Source: CAD feature listing. Evaluate the final solid. Frame: model axes, mm. Face numbers are marked on the shaded views. A direction names the side the tool comes from. Give positions to 0.01 mm unless a question says otherwise; leave off trailing zeros. Write each loop counter-clockwise with the first axis right and the second up, starting at its lowest first coordinate (ties: lowest second). Pieces come first, ordered by that corner, then holes. Notation, with made-up numbers: (48, -22) -> (104, -22) arc R23 ccw to (104, 11) -> close; hole circle Ø11 at (75, 54.25). An arc over 180 degrees is marked (long way). Write item = value, one per line.
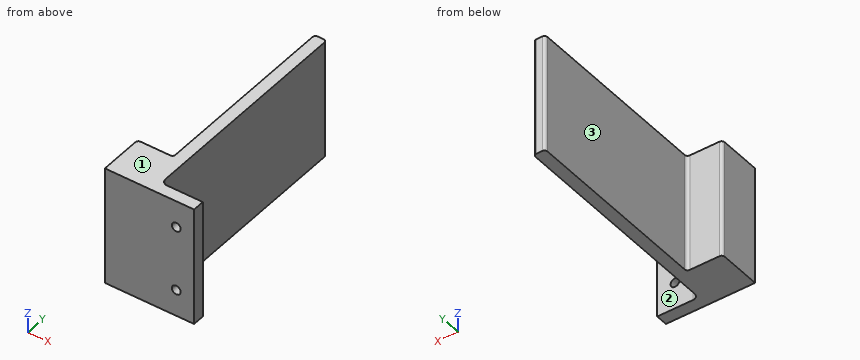
from build123d import *

# Parameters (mm, degrees)
PAD_DEPTH    = 40
FILLET_R     = 1
FILLET001_R  = 1
FILLET002_R  = 2
FILLET003_R  = 1
FILLET004_R  = 1
SKETCH001_R  = 1.5
POCKET_DEPTH = 5


with BuildPart() as part:
    # Sketch → Pad (new body)
    with BuildSketch(Plane.XY):
        Polygon((0, 0), (0, 15), (12, 15), (12, 80), (16, 80), (16, 4), (30, 4), (30, 0), align=None)
    extrude(amount=PAD_DEPTH)

    # Fillet
    fillet_edges = [part.edges().sort_by_distance(p)[0] for p in [
        (12, 80, 20),
    ]]
    fillet(fillet_edges, radius=FILLET_R)

    # Fillet001
    fillet001_edges = [part.edges().sort_by_distance(p)[0] for p in [
        (16, 80, 20),
    ]]
    fillet(fillet001_edges, radius=FILLET001_R)

    # Fillet002
    fillet002_edges = [part.edges().sort_by_distance(p)[0] for p in [
        (16, 4, 20),
    ]]
    fillet(fillet002_edges, radius=FILLET002_R)

    # Fillet003
    fillet003_edges = [part.edges().sort_by_distance(p)[0] for p in [
        (0, 15, 20),
    ]]
    fillet(fillet003_edges, radius=FILLET003_R)

    # Fillet004
    fillet004_edges = [part.edges().sort_by_distance(p)[0] for p in [
        (12, 15, 20),
    ]]
    fillet(fillet004_edges, radius=FILLET004_R)

    # Sketch001 (on Face12 of Fillet004) → Pocket (cut)
    with BuildSketch(Plane(origin=(0, 4, 0), x_dir=(-1, 0, 0), z_dir=(0, 1, 0))):
        with Locations((-24, 31)):
            Circle(SKETCH001_R)
        with Locations((-24, 9)):
            Circle(SKETCH001_R)
    extrude(amount=-POCKET_DEPTH, mode=Mode.SUBTRACT)


solid = part.part
1) Cut plane D-D (x = 9). Return the cut outline in (y, z), then the cut area to 3 significant figures.
Computed:
outline = (0, 0) -> (15, 0) -> (15, 40) -> (0, 40) -> close
area = 600 mm²
2) Material intervals for L1, parallel to Z at x = 24, y = 2.7; L2, parallel to Y at x = 20.5, z = 23.5; L3, parallel to Y at x = 7, z = 9.5, sorted ascending.
Computed:
L1 = 0 to 7.5, 10.5 to 29.5, 32.5 to 40
L2 = 0 to 4
L3 = 0 to 15
3) Cut plane B-B (z = 31). Return the cut outline in (x, y).
Computed:
outline = (0, 0) -> (22.5, 0) -> (22.5, 4) -> (18, 4) arc R2 cw to (16, 6) -> (16, 79) arc R1 ccw to (15, 80) -> (13, 80) arc R1 ccw to (12, 79) -> (12, 16) arc R1 cw to (11, 15) -> (1, 15) arc R1 ccw to (0, 14) -> close; (25.5, 0) -> (30, 0) -> (30, 4) -> (25.5, 4) -> close
4) Contact query for flat-ended pins moving along their axis: pin 1 (12 mm diameter, centred on y = 34, z = 21.5, fed in from +X); pin 2 (8 mm diameter, centred on x = 14.5, z = 13.5, fed in from -Y); pin 3 (11 mm diameter, centred on x = 5, z = 23, fed in from +Y); pin 4 (3.5 mm diameter, centred on x = 24, z = 15.5, fed in from +Y). Output: stop coordinate, or through.
Computed:
pin_1 = 16
pin_2 = 0
pin_3 = 15
pin_4 = 4
5) Cut plane A-A (x = 24). Return the cut outline in (y, z).
Computed:
outline = (0, 0) -> (4, 0) -> (4, 7.5) -> (0, 7.5) -> close; (0, 10.5) -> (4, 10.5) -> (4, 29.5) -> (0, 29.5) -> close; (0, 32.5) -> (4, 32.5) -> (4, 40) -> (0, 40) -> close
6) Cut plane C-C (y = 62). Return the cut outline in (x, z), then the cut area to 3 significant figures.
Computed:
outline = (12, 0) -> (16, 0) -> (16, 40) -> (12, 40) -> close
area = 160 mm²
7) Access query for the marked faces 1, 2 and 3. Directions: +Z, -Z, +X, -X, +Y, -Y. A direction counts if a zero-diameter tool reaches every point of the face in a straight line with its end or side. Return the directions, or none.
Computed:
face_1 = +Z, +X, -X, +Y, -Y
face_2 = +Z, -Z, +X, +Y
face_3 = +Z, -Z, -X, +Y
